from build123d import *

# Parameters (mm, degrees)
F0_R     = 3.4
F1_DEPTH = 350


# Not quite as in the source:
# - ends of sketch curves that miss each other by under 0.0002 mm in the source are joined


with BuildPart() as f1:
    # F0 (on Front) → F1 (new body)
    with BuildSketch(Plane.XZ):
        with BuildLine():
            ThreePointArc((9.0741494418, -6.7149045575), (8.0460058013, -5.1746202437), (7.685, -3.358242))
            Line((7.685, -3.358242), (7.685, 3.358242))
            ThreePointArc((7.685, 3.358242), (8.0460058013, 5.1746202437), (9.0741494418, 6.7149045575))
            Line((9.0741494418, 6.7149045575), (12.373455, 10.018326))
            ThreePointArc((12.373455, 10.018326), (12.6623276754, 10.2115396696), (13.003172, 10.279393))
            Line((13.003172, 10.279393), (15.29885, 10.279393))
            ThreePointArc((15.29885, 10.279393), (16.1968756121, 9.9074186121), (16.56885, 9.009393))
            Line((16.56885, 9.009393), (16.56885, 6.901426))
            Line((16.56885, 6.901426), (15.94, 6.901426))
            Line((15.94, 6.901426), (15.94, 5.758104))
            ThreePointArc((15.94, 5.758104), (16.3998423535, 4.6479463535), (17.51, 4.188104))
            Line((17.51, 4.188104), (18.43, 4.188104))
            ThreePointArc((18.43, 4.188104), (19.5401576465, 4.6479463535), (20, 5.758104))
            Line((20, 5.758104), (20, 16.83))
            ThreePointArc((20, 16.83), (19.0715284964, 19.0715284964), (16.83, 20))
            Line((16.83, 20), (5.63, 20))
            ThreePointArc((5.63, 20), (4.5198423535, 19.5401576465), (4.06, 18.43))
            Line((4.06, 18.43), (4.06, 17.696221))
            ThreePointArc((4.06, 17.696221), (4.5198423535, 16.5860633535), (5.63, 16.126221))
            Line((5.63, 16.126221), (6.783928, 16.126221))
            Line((6.783928, 16.126221), (6.783928, 16.886684))
            Line((6.783928, 16.886684), (9.015, 16.886684))
            ThreePointArc((9.015, 16.886684), (9.9130256121, 16.5147096121), (10.285, 15.616684))
            Line((10.285, 15.616684), (10.285, 12.922194))
            ThreePointArc((10.285, 12.922194), (10.2548511553, 12.6925072769), (10.1664472118, 12.4783818782))
            Line((10.1664472118, 12.4783818782), (6.770639, 9.078337))
            ThreePointArc((6.770639, 9.078337), (5.2289028603, 8.0471389307), (3.409789, 7.685))
            Line((3.409789, 7.685), (-3.409789, 7.685))
            ThreePointArc((-3.409789, 7.685), (-5.2289028603, 8.0471389307), (-6.7706390582, 9.0783369418))
            Line((-6.7706390582, 9.0783369418), (-10.166447, 12.478382))
            ThreePointArc((-10.166447, 12.478382), (-10.2548511553, 12.6925072769), (-10.285, 12.922194))
            Line((-10.285, 12.922194), (-10.285, 15.616684))
            ThreePointArc((-10.285, 15.616684), (-9.9130256121, 16.5147096121), (-9.015, 16.886684))
            Line((-9.015, 16.886684), (-6.783928, 16.886684))
            Line((-6.783928, 16.886684), (-6.783928, 16.126221))
            Line((-6.783928, 16.126221), (-5.63, 16.126221))
            ThreePointArc((-5.63, 16.126221), (-4.5198423535, 16.5860633535), (-4.06, 17.696221))
            Line((-4.06, 17.696221), (-4.06, 18.43))
            ThreePointArc((-4.06, 18.43), (-4.5198423535, 19.5401576465), (-5.63, 20))
            Line((-5.63, 20), (-16.83, 20))
            ThreePointArc((-16.83, 20), (-19.0715284964, 19.0715284964), (-20, 16.83))
            Line((-20, 16.83), (-20, 5.758104))
            ThreePointArc((-20, 5.758104), (-19.5401576465, 4.6479463535), (-18.43, 4.188104))
            Line((-18.43, 4.188104), (-17.51, 4.188104))
            ThreePointArc((-17.51, 4.188104), (-16.3998423535, 4.6479463535), (-15.94, 5.758104))
            Line((-15.94, 5.758104), (-15.94, 6.901426))
            Line((-15.94, 6.901426), (-16.56885, 6.901426))
            Line((-16.56885, 6.901426), (-16.56885, 9.009393))
            ThreePointArc((-16.56885, 9.009393), (-16.1968756121, 9.9074186121), (-15.29885, 10.279393))
            Line((-15.29885, 10.279393), (-13.003172, 10.279393))
            ThreePointArc((-13.003172, 10.279393), (-12.6623276754, 10.2115396696), (-12.3734550869, 10.0183259132))
            Line((-12.3734550869, 10.0183259132), (-9.07415, 6.714904))
            ThreePointArc((-9.07415, 6.714904), (-8.0460058013, 5.1746202437), (-7.685, 3.358242))
            Line((-7.685, 3.358242), (-7.685, -3.358242))
            ThreePointArc((-7.685, -3.358242), (-8.0460058013, -5.1746202437), (-9.0741494418, -6.7149045575))
            Line((-9.0741494418, -6.7149045575), (-12.373455, -10.018326))
            ThreePointArc((-12.373455, -10.018326), (-12.6623276754, -10.2115396696), (-13.003172, -10.279393))
            Line((-13.003172, -10.279393), (-15.29885, -10.279393))
            ThreePointArc((-15.29885, -10.279393), (-16.1968756121, -9.9074186121), (-16.56885, -9.009393))
            Line((-16.56885, -9.009393), (-16.56885, -6.901426))
            Line((-16.56885, -6.901426), (-15.94, -6.901426))
            Line((-15.94, -6.901426), (-15.94, -5.758104))
            ThreePointArc((-15.94, -5.758104), (-16.3998423535, -4.6479463535), (-17.51, -4.188104))
            Line((-17.51, -4.188104), (-18.43, -4.188104))
            ThreePointArc((-18.43, -4.188104), (-19.5401576465, -4.6479463535), (-20, -5.758104))
            Line((-20, -5.758104), (-20, -16.83))
            ThreePointArc((-20, -16.83), (-19.0715284964, -19.0715284964), (-16.83, -20))
            Line((-16.83, -20), (-5.63, -20))
            ThreePointArc((-5.63, -20), (-4.5198423535, -19.5401576465), (-4.06, -18.43))
            Line((-4.06, -18.43), (-4.06, -17.696221))
            ThreePointArc((-4.06, -17.696221), (-4.5198423535, -16.5860633535), (-5.63, -16.126221))
            Line((-5.63, -16.126221), (-6.783928, -16.126221))
            Line((-6.783928, -16.126221), (-6.783928, -16.886684))
            Line((-6.783928, -16.886684), (-9.015, -16.886684))
            ThreePointArc((-9.015, -16.886684), (-9.9130256121, -16.5147096121), (-10.285, -15.616684))
            Line((-10.285, -15.616684), (-10.285, -12.922194))
            ThreePointArc((-10.285, -12.922194), (-10.2548511553, -12.6925072769), (-10.1664472118, -12.4783818782))
            Line((-10.1664472118, -12.4783818782), (-6.770639, -9.078337))
            ThreePointArc((-6.770639, -9.078337), (-5.2289028603, -8.0471389307), (-3.409789, -7.685))
            Line((-3.409789, -7.685), (3.409789, -7.685))
            ThreePointArc((3.409789, -7.685), (5.2289028603, -8.0471389307), (6.7706390582, -9.0783369418))
            Line((6.7706390582, -9.0783369418), (10.166447, -12.478382))
            ThreePointArc((10.166447, -12.478382), (10.2548511553, -12.6925072769), (10.285, -12.922194))
            Line((10.285, -12.922194), (10.285, -15.616684))
            ThreePointArc((10.285, -15.616684), (9.9130256121, -16.5147096121), (9.015, -16.886684))
            Line((9.015, -16.886684), (6.783928, -16.886684))
            Line((6.783928, -16.886684), (6.783928, -16.126221))
            Line((6.783928, -16.126221), (5.63, -16.126221))
            ThreePointArc((5.63, -16.126221), (4.5198423535, -16.5860633535), (4.06, -17.696221))
            Line((4.06, -17.696221), (4.06, -18.43))
            ThreePointArc((4.06, -18.43), (4.5198423535, -19.5401576465), (5.63, -20))
            Line((5.63, -20), (16.83, -20))
            ThreePointArc((16.83, -20), (19.0715284964, -19.0715284964), (20, -16.83))
            Line((20, -16.83), (20, -5.758104))
            ThreePointArc((20, -5.758104), (19.5401576465, -4.6479463535), (18.43, -4.188104))
            Line((18.43, -4.188104), (17.51, -4.188104))
            ThreePointArc((17.51, -4.188104), (16.3998423535, -4.6479463535), (15.94, -5.758104))
            Line((15.94, -5.758104), (15.94, -6.901426))
            Line((15.94, -6.901426), (16.56885, -6.901426))
            Line((16.56885, -6.901426), (16.56885, -9.009393))
            ThreePointArc((16.56885, -9.009393), (16.1968756121, -9.9074186121), (15.29885, -10.279393))
            Line((15.29885, -10.279393), (13.003172, -10.279393))
            ThreePointArc((13.003172, -10.279393), (12.6623276754, -10.2115396696), (12.3734550869, -10.0183259132))
            Line((12.3734550869, -10.0183259132), (9.0741494418, -6.7149045575))
        make_face()
        with BuildLine():
            Line((-12.57, -18.35), (-15.55, -18.35))
            ThreePointArc((-15.55, -18.35), (-17.5298989873, -17.5298989873), (-18.35, -15.55))
            Line((-18.35, -15.55), (-18.35, -12.57))
            ThreePointArc((-18.35, -12.57), (-18.1654772721, -12.1245227279), (-17.72, -11.94))
            Line((-17.72, -11.94), (-13.21, -11.94))
            ThreePointArc((-13.21, -11.94), (-12.3119743879, -12.3119743879), (-11.94, -13.21))
            Line((-11.94, -13.21), (-11.94, -17.72))
            ThreePointArc((-11.94, -17.72), (-12.1245227279, -18.1654772721), (-12.57, -18.35))
        make_face(mode=Mode.SUBTRACT)
        with BuildLine():
            Line((13.21, -11.94), (17.72, -11.94))
            ThreePointArc((17.72, -11.94), (18.1654772721, -12.1245227279), (18.35, -12.57))
            Line((18.35, -12.57), (18.35, -15.55))
            ThreePointArc((18.35, -15.55), (17.5298989873, -17.5298989873), (15.55, -18.35))
            Line((15.55, -18.35), (12.57, -18.35))
            ThreePointArc((12.57, -18.35), (12.1245227279, -18.1654772721), (11.94, -17.72))
            Line((11.94, -17.72), (11.94, -13.21))
            ThreePointArc((11.94, -13.21), (12.3119743879, -12.3119743879), (13.21, -11.94))
        make_face(mode=Mode.SUBTRACT)
        with BuildLine():
            ThreePointArc((-17.72, 11.94), (-18.1654772721, 12.1245227279), (-18.35, 12.57))
            Line((-18.35, 12.57), (-18.35, 15.55))
            ThreePointArc((-18.35, 15.55), (-17.5298989873, 17.5298989873), (-15.55, 18.35))
            Line((-15.55, 18.35), (-12.57, 18.35))
            ThreePointArc((-12.57, 18.35), (-12.1245227279, 18.1654772721), (-11.94, 17.72))
            Line((-11.94, 17.72), (-11.94, 13.21))
            ThreePointArc((-11.94, 13.21), (-12.3119743879, 12.3119743879), (-13.21, 11.94))
            Line((-13.21, 11.94), (-17.72, 11.94))
        make_face(mode=Mode.SUBTRACT)
        Circle(F0_R, mode=Mode.SUBTRACT)
        with BuildLine():
            Line((12.57, 18.35), (15.55, 18.35))
            ThreePointArc((15.55, 18.35), (17.5298989873, 17.5298989873), (18.35, 15.55))
            Line((18.35, 15.55), (18.35, 12.57))
            ThreePointArc((18.35, 12.57), (18.1654772721, 12.1245227279), (17.72, 11.94))
            Line((17.72, 11.94), (13.21, 11.94))
            ThreePointArc((13.21, 11.94), (12.3119743879, 12.3119743879), (11.94, 13.21))
            Line((11.94, 13.21), (11.94, 17.72))
            ThreePointArc((11.94, 17.72), (12.1245227279, 18.1654772721), (12.57, 18.35))
        make_face(mode=Mode.SUBTRACT)
    extrude(amount=F1_DEPTH)


solid = f1.part
Could you check a few things on this model? Use its own coordinates, in mm. A direction names the side the tool comes from. Coordinates: 2 decimals unless noted, no trailing zeros. Write each loop counter-clockwise with the first axis right and the second up, starting at its lowest first coordinate (ties: lowest second). Pieces come first, ordered by that corner, then holes. Notation, with made-up numbers: (-29.75, -7.75) - (-3.75, -7.75) arc R13 ccw to (-3.75, 3.25) - close; hole circle Ø3 at (6, 74.5). An arc over 180 degrees is marked (long way). Put each result on its own line as item: value. Start each with the question number.
Q1. Please list where these lines run through material, in increasing order: L1, parallel to Z at x = 17.5, y = -64; L2, parallel to X at y = -82.5, z = 7; L3, parallel to Z at x = 0, y = -100.5 (3 decimals).
Q2. I want a section at A-A on z = 0. Write out the boundary of the cut face in (x, y) (3 decimals), plus the area to 3 significant figures.
Q3. I want a section at C-C on y = -169.5. Count the separate pieces of the cut face and the enclosed holes in it, plus the area to 3 significant figures.
Q4. I want a section at B-B on x = 0. Write out the boundary of the cut face in (y, z) (3 decimals).
Q5. I'm going to push flat-ended pins straight in: P1, Ø5.5, axis at x = -0.5, y = -251.5, coming from the -Z side (3 decimals); P2, Ø10, axis at y = -85, z = 0, coming from the +X side. Where does each tip first touch, or does it pass through?
Q6. Which directions (+Z, -Z, +X, -X, +Y, -Y) give clear straight access to the entire face, cutting with the end or side of a thin tool? Please do faces 1 (the flat face through (-7.685, -173, 0)), 2 (the flat face through (7.685, -173, 0)), 3 (the flat face through (20, -173, -11)), 4 (the flat face through (0, -173, -7.685)), 5 (the flat face through (0, -173, 7.685)).
Q7. Thinking about a two-plate mould opening in X: for faces 6 (the cylindrical face through (-0.74, -172.55, -3.32)), 7 (the flat face through (11, -173, -20)), 8 (the flat face through (20, -173, 11)), which applies, pulls with the +X half, pulls with the -X half, needs draft (parallel to the pull), parting line crosses it, or undercut?
Checks:
1. L1: -19.93 to -17.56, -11.94 to -4.19, 4.19 to 11.94, 17.56 to 19.93
1. L2: -20 to -16.57, -9.36 to 9.36, 16.57 to 20
1. L3: -7.685 to -3.4, 3.4 to 7.685
2. outline: (-7.685, -350) - (-3.4, -350) - (-3.4, 0) - (-7.685, 0) - close; (3.4, -350) - (7.685, -350) - (7.685, 0) - (3.4, 0) - close
2. area: 3,000 mm²
3. separate pieces: 1
3. enclosed holes: 5
3. area: 658 mm²
4. outline: (-350, -7.685) - (0, -7.685) - (0, -3.4) - (-350, -3.4) - close; (-350, 3.4) - (0, 3.4) - (0, 7.685) - (-350, 7.685) - close
5. P1: z = -7.685
5. P2: x = 19.8
6. face 1: -X, +Y, -Y
6. face 2: +X, +Y, -Y
6. face 3: +Z, -Z, +X, +Y, -Y
6. face 4: -Z, +Y, -Y
6. face 5: +Z, +Y, -Y
7. face 6: undercut
7. face 7: needs draft
7. face 8: pulls with the +X half
